Source: CAD feature listing. Evaluate the final solid. Frame: model axes, mm. A direction names the side the tool comes from. Give positions to 0.01 mm unless a question says otherwise; leave off trailing zeros. Order: outer loops, then holes, each group sorted by start corner. A loop starts at its lowest first (then second) coordinate and runs counter-clockwise, first axis right, second up. Notation, with made-up numbers: (-21, 62.25) -> (-10, 62.25) arc R16 cw to (-10, 74.25) -> close; hole circle Ø9 at (9, 69.25). An arc over 180 degrees is marked (long way). Use CSV: the item, a comma, the result in double quotes.
Autodesk Inventor part; units mm, degrees
ref_plane "Work Plane1" through (6.25, 0, 0) normal (-1, 0, 0) x (0, 0, 1)
ref_plane "YZ Plane" through (0, 0, 0) normal (1, 0, 0) x (0, 1, 0)
ref_plane "XZ Plane" through (0, 0, 0) normal (0, 1, 0) x (-1, 0, 0)
sketch "Sketch1" plane through (0, 0, 0) normal (1, 0, 0) x (0, 1, 0)
  circle A0 centre (0, 0) radius 12.5
  dimension "d0" = 25
extrude "Extrusion1" add sketch "Sketch1" along normal blind 12.5
ref_plane "Work Plane1" through (6.25, 0, 0) normal (-1, 0, 0) x (0, 0, 1)
sketch "Sketch2" plane through (12.5, 0, 0) normal (1, 0, 0) x (0, 0, -1)
  circle A0 centre (0, 0) radius 6
  dimension "d3" = 12
extrude "Extrusion2" add sketch "Sketch2" along normal blind 2.5
fillet "Fillet1" radius 2.5 1 edges at (15, 0, 6)
sketch "Sketch3" plane through (15, 0, 0) normal (1, 0, 0) x (0, 0, -1)
  circle A0 centre (0, 0) radius 7.5
  line L0 (-21.125, -11) -> (21.125, -11)
  line L1 (21.125, -11) -> (21.125, -16)
  line L2 (21.125, -16) -> (-21.125, -16)
  line L3 (-21.125, -16) -> (-21.125, -11)
  line L4 (-7.5, 0) -> (7.5, 0)
  line L5 (7.5, 0) -> (7.5, -11)
  line L6 (7.5, -11) -> (-7.5, -11)
  line L7 (-7.5, -11) -> (-7.5, 0)
  line L8 (6, -16) -> (-6, -16)
  line L9 (-6, -16) -> (-6, -14.75)
  line L10 (-6, -14.75) -> (6, -14.75)
  line L11 (6, -14.75) -> (6, -16)
  dimension "d7" = 15
  dimension "d8" = 16
  dimension "d9" = 5
  dimension "d10" = 42.25
  dimension "d11" = 21.125
  dimension "d21" = 12
  dimension "d22" = 6
  dimension "d23" = 1.25
extrude "Extrusion3" add sketch "Sketch3" along normal blind 1.25 contours L4 A0 | L5 L0 L7 A0 | A0 L4 | L0 L1 L2 L11 L10 L9 L3
fillet "Fillet2" radius 14 2 edges at (15.625, -11, -7.5) (15.625, -11, 7.5)
fillet "Fillet3" radius 2 2 edges at (15.625, -10.999, 21.125) (15.625, -10.999, -21.125)
sketch "Sketch5" plane through (16.25, 0, 0) normal (1, 0, 0) x (0, 0, -1)
  circle A0 centre (0, 0) radius 4.265
  dimension "d25" = 8.53
extrude "Extrusion5" add sketch "Sketch5" along normal blind 2.17
fillet "Fillet5" radius 1.5 1 edges at (18.42, 0, 4.265)
mirror "Mirror1" about plane through (6.25, 0, 0) normal (-1, 0, 0) of "Extrusion2", "Fillet1", "Extrusion3", "Fillet2", "Fillet3", "Extrusion5", "Fillet5"
sketch "Sketch4" plane through (-2.5, -16, 21.125) normal (1, 0, 0) x (0, 0, -1)
  line L0 (0, 0) -> (42.25, 0)
  line L1 (42.25, 0) -> (27.125, 0)
  line L2 (27.125, 0) -> (27.125, 1.25)
  line L3 (27.125, 1.25) -> (42.25, 1.25)
  line L4 (42.25, 1.25) -> (42.25, 0)
  line L5 (0, 0) -> (42.25, 0)
  line L6 (0, 0) -> (15.125, 0)
  line L7 (15.125, 0) -> (15.125, 1.25)
  line L8 (15.125, 1.25) -> (0, 1.25)
  line L9 (0, 1.25) -> (0, 0)
  point P0 (21.125, 16)
  point P1 (15.125, 0)
  point P2 (27.125, 0)
  point P3 (27.125, 1.25)
  point P4 (15.125, 1.25)
  dimension "d16" = 1.25
extrude "Extrusion4" add sketch "Sketch4" along normal up to surface (17.5 mm away)
fillet "Fillet4" radius 1.25 4 edges at (-3.75, -16, -13.5625) (16.25, -16, -13.5625) (16.25, -16, 13.5625) (-3.75, -16, 13.5625)
sketch "Sketch6" plane through (-2.5, -16, 6) normal (0, -1, 0) x (1, 0, 0)
  line L0 (0, 15.125) -> (17.5, 15.125)
  point P0 (2.5, -6)
  point P1 (8.75, 10)
  point P2 (8.75, -22)
  point P3 (8.75, 15.125)
  dimension "d29" = 32
  dimension "d30" = 16
hole "Hole1" at (6.25, -16, 16) at (6.25, -16, -16) direction (0, 1, 0) diameter 4 end through all
properties part number "caster_d25"
1. Section query C-C on x = 9.5. Return loops of the section in (y, z) (3 decimals).
Answer below:
outline,"(-16, -21.125) -> (-14.75, -21.125) -> (-14.75, -6) -> (-16, -6) -> close; (-16, 6) -> (-14.75, 6) -> (-14.75, 21.125) -> (-16, 21.125) -> close; circle Ø25 at (0, 0)"
2. Ray query, line 1 along Z through (x, y) = (6.25, -15.15) (3 decimals); line 2 along X through (y, z) = (-9, -2.5); line 3 along X through (y, z) = (-12, 8). Return the intervals inside material, ascending.
Answer below:
line 1,"z = -21.125 to -18, -14 to -6, 6 to 14, 18 to 21.125"
line 2,"x = -3.75 to -2.5, 0 to 12.5, 15 to 16.25"
line 3,"x = -3.75 to -2.5, 15 to 16.25"
3. Access query for faces 1 (the flat face through (6, -14.75, 13)), 2 (the cylindrical face through (-3.12, -7.01, 11.5)), 3 (the cylindrical face through (16.58, 4.164, 0.925)), 4 (the flat face through (-3, -14.75, 0)), 5 (the cylindrical face through (6.162, 11.923, -3.755)). Directions: +Z, -Z, +X, -X, +Y, -Y. A direction counts if a zero-diameter tool reaches every point of the face in a straight line with its end or side. Return the directions, or none.
Answer below:
face 1,"+Z, -Z"
face 2,"+Z, -X, +Y"
face 3,"+X"
face 4,"+X, -X, -Y"
face 5,"none"
4. Section query A-A on z = -14.5. Return loops of the section in (x, y).
Answer below:
outline,"(-3.75, -14.75) arc R1.25 ccw to (-2.5, -16) -> (4.93, -16) -> (4.93, -14.75) -> (-2.5, -14.75) -> (-2.5, -9.24) -> (-3.75, -9.24) -> close; (7.57, -16) -> (15, -16) arc R1.25 ccw to (16.25, -14.75) -> (16.25, -9.24) -> (15, -9.24) -> (15, -14.75) -> (7.57, -14.75) -> close"
5. Section query B-B on y = -8. Return loops of the section in (x, z), plus the area to 3 significant figures.
Answer below:
outline,"(-3.75, -12.63) -> (-2.5, -12.63) -> (-2.5, 12.63) -> (-3.75, 12.63) -> close; (0, -9.6) -> (12.5, -9.6) -> (12.5, 9.6) -> (0, 9.6) -> close; (15, -12.63) -> (16.25, -12.63) -> (16.25, 12.63) -> (15, 12.63) -> close"
area,"303 mm²"
6. Mould query, pull axis X, two halves, no side actions, for faces 6 (the flat face through (0, -3, -5.4)), 7 (the cylindrical face through (15.874, -15.644, -13.457)), 8 (the cylindrical face through (15.62, -7.01, -11.5)). Classes: released by +X, released by -X, zero draft, split by the parting line, or undercut.
Answer below:
face 6,"undercut"
face 7,"released by +X"
face 8,"zero draft"
7. Section query D-D on y = 9. Return loops of the section in (x, z).
Answer below:
outline,"(0, -8.67) -> (12.5, -8.67) -> (12.5, 8.67) -> (0, 8.67) -> close"
8. Pin query (flat end, axial travel): P1, Ø4, axis at y = 4.5, z = 11.5, coming from the -X side; P2, Ø1.4, axis at x = -3, z = -1.5, coming from the -Y side; P3, Ø8, axis at y = -12, z = -11.5, coming from the -X side; P4, Ø2.5, axis at x = 6.25, z = -16, coming from the -Y side. Return the tip coordinate at first contact, or that it passes through.
Answer below:
P1,"stops at x = 0"
P2,"stops at y = -14.75"
P3,"stops at x = -3.75"
P4,"passes through"
